Build history of the part. All positions in model axes, mm. A direction names the side the tool comes from. Coordinates: 2 decimals unless noted, no trailing zeros. Loops run counter-clockwise (first coordinate to the right, second up) from the corner with the lowest first, then second, coordinate; pieces in that order, holes last. Notation, with made-up numbers: (41.5, 83.25) - (52.5, 83.25) arc R10 ccw to (52.5, 90.25) - close; hole circle Ø4 at (48.5, -21). An arc over 180 degrees is marked (long way). One line per item, written item: value.
```python
from build123d import *

# Parameters (mm, degrees)
F1_DEPTH = 70.358
F2_W     = 70.358
F2_H     = 20.955
F3_DEPTH = 65.532
F4_W     = 64.008
F4_H     = 17.78
F5_DEPTH = 93.472


with BuildPart() as f1:
    # F0 (on Front) → F1 (new body)
    with BuildSketch(Plane.XZ):
        with BuildLine():
            ThreePointArc((0, -19.731941), (-8.27847, -11.45347), (0, -3.175))
            Line((0, -3.175), (84, -3.175))
            Line((84, -3.175), (84, 0))
            Line((84, 0), (0, 0))
            ThreePointArc((0, 0), (-11.45347, -11.45347), (0, -22.906941))
            Line((0, -22.906941), (0, -19.731941))
        make_face()
    extrude(amount=F1_DEPTH)

    # F2 (on face) → F3 (join)
    with BuildSketch(Plane.YZ.offset(84)):
        with Locations((-35.179, 10.4775)):
            Rectangle(F2_W, F2_H)
    extrude(amount=-F3_DEPTH)

    # F4 (on face) → F5 (cut)
    with BuildSketch(Plane.YZ.offset(84)):
        with Locations((-35.179, 8.89)):
            Rectangle(F4_W, F4_H)
    extrude(amount=-F5_DEPTH, mode=Mode.SUBTRACT)


solid = f1.part
```
Item 1: Cut at D-D, the plane z = -8.5. Write the cut outline in (x, y).
Check result:
outline: (-11.07, -70.36) - (-7.73, -70.36) - (-7.73, 0) - (-11.07, 0) - close
Item 2: Drop flat-ended pins along their axis: P1, Ø6, axis at x = 32.5, y = -52, coming from the -Z side (3 decimals); P2, Ø10.5, axis at y = -47, z = 7.5, coming from the -X side; P3, Ø14, axis at x = 50.5, z = 4.5, coming from the +Y side; P4, Ø1.6, axis at y = -21.5, z = -22, coming from the +X side. Give the stop position or say it passes through.
Check result:
P1: stops at z = -3.175
P2: passes through
P3: stops at y = 0
P4: stops at x = 0
Item 3: Tool access for faces 1 (the face through (18.468, -35, 18)), 2 (the face through (0, -35, -21)), 3 (the face through (52, -67.183, 9)), 4 (the face through (-11.45, -34.69, -11.2)), 5 (the face through (48, 0, 8)): list every direction of +Z, -Z, +X, -X, +Y, -Y with a clear straight run to the whole face (end or side of a thin tool).
Check result:
face 1: +Z, -X, +Y, -Y
face 2: -Z, +X, +Y, -Y
face 3: +X, -X
face 4: -X, +Y, -Y
face 5: +Z, -Z, +X, -X, +Y
Item 4: Cut at B-B, the plane y = -52. Write the cut outline in (x, z) (3 decimals), then the cut area to 3 significant figures.
Check result:
outline: (0, -22.907) - (0, -19.732) arc R8.278 cw to (0, -3.175) - (84, -3.175) - (84, 0) - (0, 0) arc R11.453 ccw to start; (18.468, 17.78) - (84, 17.78) - (84, 20.955) - (18.468, 20.955) - close
area: 573 mm^2
Item 5: Cut at A-A, the plane x = 46. Write the cut outline in (y, z) (3 decimals).
Check result:
outline: (-70.358, -3.175) - (0, -3.175) - (0, 20.955) - (-70.358, 20.955) - close; hole (-67.183, 0) - (-3.175, 0) - (-3.175, 17.78) - (-67.183, 17.78) - close
Item 6: Probe probe 1 along Z at (x, y) = (68.5, -48.5) (3 decimals); probe 2 along Y at (x, z) = (74.5, 3) (3 decimals); probe 3 along Z at (x, y) = (-0.5, -27.5). List the from-to ranges inside material, lowest first. Write a range as from..to.
Check result:
probe 1: z = -3.175..0, 17.78..20.955
probe 2: y = -70.358..-67.183, -3.175..0
probe 3: z = -22.9..-19.72, -3.19..-0.01
Item 7: Pull direction Y, two halves, no side cores. Call faces 6 (the face through (52, -36, 17.78)), 7 (the face through (52, -3.175, 9)), 8 (the face through (48, -70.358, 8)), 9 (the face through (84, -38, 18)): released by +Y, released by -Y, zero draft, split by the parting line, or undercut.
Check result:
face 6: undercut
face 7: undercut
face 8: released by -Y
face 9: zero draft
Item 8: Cut at C-C, the plane z = -1.5. Write the cut outline in (x, y).
Check result:
outline: (-5.67, -70.36) - (84, -70.36) - (84, 0) - (-5.67, 0) - close
